The listing builds one solid part. Answer for the finished solid, in the listing's coordinates (mm). A direction names the side the tool comes from. Coordinates: 2 decimals unless noted, no trailing zeros. Order: outer loops, then holes, each group sorted by start corner. A loop starts at its lowest first (then second) coordinate and runs counter-clockwise, first axis right, second up. Notation, with made-up numbers: (-21, 4) -> (1, 4) arc R17 cw to (1, 23) -> close; hole circle Ø3 at (-8, -26.5). An arc over 180 degrees is marked (long way). Return JSON: item names as keys, results as strings.
from build123d import *
from build123d.topology import SkipClean

# Parameters (mm, degrees)
SKETCH1_W           = 26
SKETCH1_H           = 15
BOSS_EXTRUDE1_DEPTH = 15
SKETCH2_R           = 1.5
CUT_EXTRUDE1_DEPTH  = 22.219095174
SKETCH3_R           = 7
BOSS_EXTRUDE2_DEPTH = 8
BOSS_EXTRUDE3_DEPTH = 7.5
SKETCH5_R           = 5
BOSS_EXTRUDE4_DEPTH = 13
BOSS_EXTRUDE5_START = 5
SKETCH6_R           = 7
BOSS_EXTRUDE5_DEPTH = 5
BOSS_EXTRUDE6_START = 12.5
BOSS_EXTRUDE6_DEPTH = 12.5
DOME1_FACE_RADIUS   = 5
DOME1_HEIGHT        = 1.3


with BuildPart() as part:
    # Sketch1 → Boss-Extrude1 (new body)
    with BuildSketch(Plane(origin=(0, 0, 0), x_dir=(1, 0, 0), z_dir=(0, 1, 0))):
        Rectangle(SKETCH1_W, SKETCH1_H)
    extrude(amount=BOSS_EXTRUDE1_DEPTH)

    # Sketch2 → Cut-Extrude1 (cut, through all)
    with BuildSketch(Plane(origin=(0, 15, 0), x_dir=(1, 0, 0), z_dir=(0, 1, 0))):
        with Locations(Location((-7, 0, 0), (0, 0, 270))):
            Circle(SKETCH2_R)
    extrude(amount=-CUT_EXTRUDE1_DEPTH, mode=Mode.SUBTRACT)

    # Sketch3 → Boss-Extrude2 (add)
    with BuildSketch(Plane.ZY.offset(13)):
        with Locations((0, 7.5)):
            Circle(SKETCH3_R)
    extrude(amount=BOSS_EXTRUDE2_DEPTH)

    # Sketch4 → Boss-Extrude3 (add)
    with BuildSketch(Plane.ZY.offset(21)):
        with BuildLine():
            Line((4.898979486, 12.5), (-4.898979486, 12.5))
            ThreePointArc((-4.898979486, 12.5), (-4.949747468, 12.449747468), (-5, 12.398979486))
            Line((-5, 12.398979486), (-5, 2.601020514))
            ThreePointArc((-5, 2.601020514), (-4.949747468, 2.550252532), (-4.898979486, 2.5))
            Line((-4.898979486, 2.5), (4.898979486, 2.5))
            ThreePointArc((4.898979486, 2.5), (4.949747468, 2.550252532), (5, 2.601020514))
            Line((5, 2.601020514), (5, 12.398979486))
            ThreePointArc((5, 12.398979486), (4.949747468, 12.449747468), (4.898979486, 12.5))
        make_face()
    extrude(amount=BOSS_EXTRUDE3_DEPTH)

    # Sketch5 → Boss-Extrude4 (add)
    with BuildSketch(Plane.ZY.offset(28.5)):
        with Locations((0, 7.5)):
            Circle(SKETCH5_R)
    extrude(amount=BOSS_EXTRUDE4_DEPTH)

    # Sketch6 → Boss-Extrude5 (add)
    with BuildSketch(Plane(origin=(13, 0, 0), x_dir=(0, 0, -1), z_dir=(1, 0, 0)).offset(BOSS_EXTRUDE5_START)):
        with Locations(Location((0, 7.5, 0), (0, 0, 315.584691403))):
            Circle(SKETCH6_R)
    extrude(amount=-BOSS_EXTRUDE5_DEPTH)

    # Sketch7 → Boss-Extrude6 (add)
    with SkipClean():  # the faces are left unmerged after this step: merging them gives an invalid solid
        with BuildSketch(Plane(origin=(18, 0, 0), x_dir=(0, 0, -1), z_dir=(1, 0, 0)).offset(BOSS_EXTRUDE6_START)):
            with BuildLine():
                ThreePointArc((-5, 2.601020514), (-4.949747468, 2.550252532), (-4.898979486, 2.5))
                Line((-4.898979486, 2.5), (4.898979486, 2.5))
                ThreePointArc((4.898979486, 2.5), (4.949747468, 2.550252532), (5, 2.601020514))
                Line((5, 2.601020514), (5, 12.398979486))
                ThreePointArc((5, 12.398979486), (4.949747468, 12.449747468), (4.898979486, 12.5))
                Line((4.898979486, 12.5), (-4.898979486, 12.5))
                ThreePointArc((-4.898979486, 12.5), (-4.949747468, 12.449747468), (-5, 12.398979486))
                Line((-5, 12.398979486), (-5, 2.601020514))
            make_face()
        extrude(amount=-BOSS_EXTRUDE6_DEPTH)

    # Dome1: a dome of height H over a round flat face of radius A is a cap of a sphere of radius (A * A + H * H) / (2 * H)
    dome1_r = (DOME1_FACE_RADIUS * DOME1_FACE_RADIUS + DOME1_HEIGHT * DOME1_HEIGHT) / (2 * DOME1_HEIGHT)
    dome1_base = Plane((-41.5, 7.5, 0), z_dir=(-1, 0, 0))
    with Locations(dome1_base.offset(DOME1_HEIGHT - dome1_r)):
        dome1_ball = Sphere(dome1_r, mode=Mode.PRIVATE)
    add(split(dome1_ball, bisect_by=dome1_base, keep=Keep.TOP, mode=Mode.PRIVATE))


solid = part.part
1. Each of these flat-tipped pins is pushed along its axis until it touches: pin 1 Ø3 at (x, z) = (25, 2) entering from -Y; pin 2 Ø4 at (x, y) = (-26, 8.5) entering from +Z; pin 3 Ø1.5 at (x, z) = (17.5, 3.5) entering from +Y. Where does it stop, or does it pass through?
Answer block:
{"pin 1": "stops at y = 2.5", "pin 2": "stops at z = 5", "pin 3": "stops at y = 13.94"}
2. For faces 1 (the face through (18, 2, 0)), 2 (the face through (-13, 10, 7)), 3 (the face through (18, 7, 6)), determine the directions among +Z, -Z, +X, -X, +Y, -Y from which every point of the face is accessible in a straight line to the end or side of a thin tool.
Answer block:
{"face 1": "+Z, -Z, +X, -Y", "face 2": "-X", "face 3": "+Z, +X, +Y, -Y"}
3. Consider line 1 (X direction, y = 14, z = -1.75); line 2 (X direction, y = 11.5, z = -6.5); line 3 (X direction, y = 8, z = 0). Determine where each line is inside the solid, lowest interval first. Write a range as from..to.
Answer block:
{"line 1": "x = -21..18", "line 2": "x = -13..13", "line 3": "x = -42.79..-8.5, -5.5..30.5"}
4. The part is cut by section A-A on x = -7. Give the vertices of the cut face in (y, z), and give its area (3 significant figures).
Answer block:
{"outline": "(0, -7.5) -> (15, -7.5) -> (15, -1.5) -> (0, -1.5) -> close; (0, 1.5) -> (15, 1.5) -> (15, 7.5) -> (0, 7.5) -> close", "area": "180 mm2"}
5. The part is cut by section C-C on x = 14. Give the vertices of the cut face in (y, z).
Answer block:
{"outline": "circle Ø14 at (7.5, 0)"}
6. The part is cut by section B-B on y = 3.5. Give the vertices of the cut face in (x, z), and give its area (3 significant figures).
Answer block:
{"outline": "(-41.5, -3) -> (-28.5, -3) -> (-28.5, -5) -> (-21, -5) -> (-21, -5.74) -> (-13, -5.74) -> (-13, -7.5) -> (13, -7.5) -> (13, -5.74) -> (18, -5.74) -> (18, -5) -> (30.5, -5) -> (30.5, 5) -> (18, 5) -> (18, 5.74) -> (13, 5.74) -> (13, 7.5) -> (-13, 7.5) -> (-13, 5.74) -> (-21, 5.74) -> (-21, 5) -> (-28.5, 5) -> (-28.5, 3) -> (-41.5, 3) arc R9.45 ccw to start; hole circle Ø3 at (-7, 0)", "area": "812 mm2"}
